Build history of the part. All positions in model axes, mm. Face numbers are marked on the shaded views. A direction names the side the tool comes from. Give positions to 0.01 mm unless a question says otherwise; leave off trailing zeros. Write each loop counter-clockwise with the first axis right and the second up, starting at its lowest first coordinate (ties: lowest second). Pieces come first, ordered by that corner, then holes. Notation, with made-up numbers: (35.5, 43) -> (88.5, 43) arc R17 ccw to (88.5, 48) -> close; hole circle Ø6 at (9, 67.5). An arc over 180 degrees is marked (long way). Write item = value, one per line. Start each with the question number.
Q1. Wall check: line 1 (Z direction, x = 13.1, y = 2.75); line 2 (X direction, y = 3, z = -63); line 3 (Y direction, x = 28, z = -7). Give the ranges that are in metal, low to high.
Q2. Tool access for the marked faces 1 and 2: list every direction of +Z, -Z, +X, -X, +Y, -Y with a clear straight run to the whole face (end or side of a thin tool).
Q3. Drop flat-ended pins along their axis: P1, Ø5, axis at x = 51.5, z = -9.5, coming from the -Y side; P2, Ø10, axis at x = 51, y = 314.5, coming from the +Z side; P3, Ø1.5, axis at x = 41, y = 62, coming from the +Z side; P4, Ø8, axis at y = 74.5, z = -16.5, coming from the -X side. Give the stop position or say it passes through.
Q4. Saw through at B-B, the plane z = -38.1. List the corners of the cut face in (x, y), then the cut area to 3 significant figures.
Q5. Saw through at C-C, the plane y = 49. List the corners of the cut face in (x, z), then the cut area to 3 significant figures.
Q6. Saw through at A-A, the plane x = 38.1. List the corners of the cut face in (y, z).
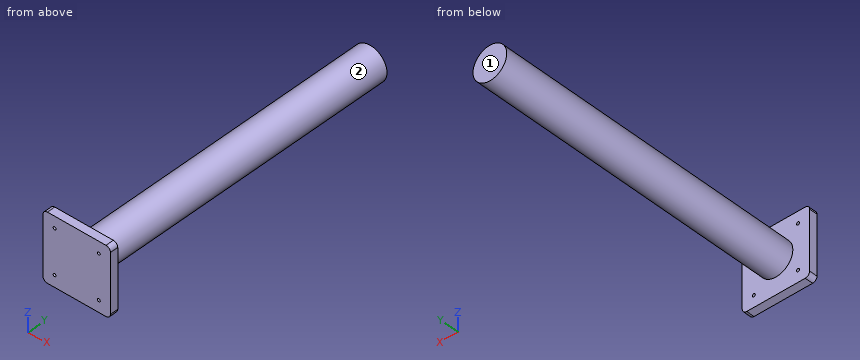
from build123d import *

# Parameters (mm, degrees)
SKETCH1_W           = 76.2
SKETCH1_H           = 76.2
BOSS_EXTRUDE1_DEPTH = 9.144
SKETCH2_R           = 1.65
CUT_EXTRUDE1_DEPTH  = 9.144
SKETCH3_R           = 19.05
BOSS_EXTRUDE2_DEPTH = 355.6
FILLET1_R           = 5


with BuildPart() as part:
    # Sketch1 → Boss-Extrude1 (new body)
    with BuildSketch(Plane(origin=(0, 0, 0), x_dir=(1, 0, 0), z_dir=(0, 1, 0))):
        with Locations((38.1, 38.1)):
            Rectangle(SKETCH1_W, SKETCH1_H)
    extrude(amount=BOSS_EXTRUDE1_DEPTH)

    # Sketch2 → Cut-Extrude1 (cut)
    with BuildSketch(Plane(origin=(0, 9.144, 0), x_dir=(1, 0, 0), z_dir=(0, 1, 0))):
        with Locations((13.1, 63.1)):
            Circle(SKETCH2_R)
        with Locations((63.1, 63.1)):
            Circle(SKETCH2_R)
        with Locations((63.1, 13.1)):
            Circle(SKETCH2_R)
        with Locations((13.1, 13.1)):
            Circle(SKETCH2_R)
    extrude(amount=-CUT_EXTRUDE1_DEPTH, mode=Mode.SUBTRACT)

    # Sketch3 → Boss-Extrude2 (add)
    with BuildSketch(Plane(origin=(0, 9.144, 0), x_dir=(1, 0, 0), z_dir=(0, 1, 0))):
        with Locations((38.1, 38.1)):
            Circle(SKETCH3_R)
    extrude(amount=BOSS_EXTRUDE2_DEPTH)

    # Fillet1
    fillet1_edges = [part.edges().sort_by_distance(p)[0] for p in [
        (0, 4.572, -76.2),
        (76.2, 4.572, -76.2),
        (76.2, 4.572, 0),
        (0, 4.572, 0),
    ]]
    fillet(fillet1_edges, radius=FILLET1_R)


solid = part.part
Report:
q1.line_1 = -76.2 to -64.75, -61.45 to -14.75, -11.45 to 0
q1.line_2 = 0 to 11.45, 14.75 to 61.45, 64.75 to 76.2
q1.line_3 = 0 to 9.14
q2.face_1 = +Z, -Z, +X, -X, +Y
q2.face_2 = +Y
q3.P1 = 0
q3.P2 = -20.77
q3.P3 = -19.17
q3.P4 = 30.81
q4.outline = (0, 0) -> (76.2, 0) -> (76.2, 9.14) -> (57.15, 9.14) -> (57.15, 364.74) -> (19.05, 364.74) -> (19.05, 9.14) -> (0, 9.14) -> close
q4.area = 14,200 mm2
q5.outline = circle Ø38.1 at (38.1, -38.1)
q5.area = 1,140 mm2
q6.outline = (0, -76.2) -> (9.14, -76.2) -> (9.14, -57.15) -> (364.74, -57.15) -> (364.74, -19.05) -> (9.14, -19.05) -> (9.14, 0) -> (0, 0) -> close
